The model under review builds one solid part; all positions refer to its coordinate system, in mm. A direction names the side the tool comes from. Coordinates: 2 decimals unless noted, no trailing zeros. Order: outer loops, then holes, each group sorted by start corner. A loop starts at its lowest first (then second) coordinate and runs counter-clockwise, first axis right, second up. Notation, with made-up numbers: M 74,-20.75 L 104,-20.75 A36 ccw 104,15.25 Z; hole C 83,63.25 d4. An arc over 180 degrees is marked long. Answer in a Markdown table with one row per item.
from build123d import *

# Parameters (mm, degrees)
F2_R     = 2.38125
F3_DEPTH = 25.4
F4_R     = 6.35
F5_DEPTH = 15.621
F6_R     = 5.5626
F7_DEPTH = 6.35


with BuildPart() as f1:
    # F0 (on Front) → F1 (revolve)
    with BuildSketch(Plane.XZ):
        Polygon((-535.686, 0), (14.986, 0), (14.986, 6.35), (0, 6.35), (0, 7.9375), (-520.7, 7.9375), (-520.7, 6.35), (-535.686, 6.35), align=None)
    revolve(axis=Axis((-260.35, 0, 0), (1, 0, 0)))

    # F2 (on Top) → F3 (cut, symmetric)
    with BuildSketch(Plane.XY):
        with Locations((6.35, 0)):
            Circle(F2_R)
        with Locations((-527.05, 0)):
            Circle(F2_R)
    extrude(amount=F3_DEPTH, both=True, mode=Mode.SUBTRACT)

    # F4 (on Top) → F5 (join)
    with BuildSketch(Plane.XY):
        with Locations((-336.55, 0)):
            Circle(F4_R)
        with Locations((-184.15, 0)):
            Circle(F4_R)
    extrude(amount=-F5_DEPTH)

    # F6 (on face) → F7 (join)
    with BuildSketch(Plane(origin=(0, 0, -15.621), x_dir=(1, 0, 0), z_dir=(0, 0, -1))):
        with Locations((-336.55, 0)):
            Circle(F6_R)
        with Locations((-184.15, 0)):
            Circle(F6_R)
    extrude(amount=F7_DEPTH)


solid = f1.part
(1) Machinability: for faces 4 (the cylindrical face through (-181.22, -5.634, -11.322)), 5 (the cylindrical face through (7.388, 2.432, 5.866)), 6 (the cylindrical face through (-263.99, 7.75, -1.72)), which of the approach directions +Z, -Z, +X, -X, +Y, -Y give a long, thin tool a straight path to every point of the face, cutting with its end or side? Answer none if there is none.
Report:
| item | result |
|---|---|
| face 4 | -Z |
| face 5 | +X |
| face 6 | none |
(2) The part is to be moulded in two halves that separate along X. For faces 1 (the flat face through (-337, 0, -21.971)), 2 (the flat face through (-184, -6, -15.621)), 3 (the flat face through (-535.686, 0, 0)), say which applies: +X half, -X half, draft (parallel to the pull), parting line (faces both ways), or undercut.
Report:
| item | result |
|---|---|
| face 1 | draft |
| face 2 | undercut |
| face 3 | -X half |
(3) Insertion check: P1, Ø1, axis at x = -435, z = 1.5, coming from the -Y side; P2, Ø2, axis at y = 4, z = -7, coming from the -X side; P3, Ø5.5, axis at x = -527.05, y = 0, coming from the +Z side; P4, Ø4.5, axis at x = 6.35, y = 0, coming from the +Z side. Each pin has a flat end and moves straight along its axis. Give the tip position at first contact, or say it passes through.
Report:
| item | result |
|---|---|
| P1 | y = -7.87 |
| P2 | x = -520.7 |
| P3 | z = 6.35 |
| P4 | through |
(4) Take a section at C-C (x = -419). Write out the cut boundary in (y, z) (1 decimal).
Report:
| item | result |
|---|---|
| outline | C 0,0 d15.9 |
(5) To check wall thickness, follow line 1 (X direction, y = 0, z = 2); line 2 (Y direction, x = 6.35, z = -3.25); line 3 (Y direction, x = -527.05, z = 0.5). State the ranges of each line that lie inside material, in increasing order. Write a range as [from, to].
Report:
| item | result |
|---|---|
| line 1 | [-535.69, -529.43], [-524.67, 3.97], [8.73, 14.99] |
| line 2 | [-5.46, -2.38], [2.38, 5.46] |
| line 3 | [-6.33, -2.38], [2.38, 6.33] |
(6) Take a section at A-A (y = 0). State how many separate pieces and enclosed holes the cut face has, then the cut area to 3 significant figures.
Report:
| item | result |
|---|---|
| separate pieces | 3 |
| enclosed holes | 0 |
| area | 8,860 mm^2 |
